Geometry check sheet. Reference: the model listing, model coordinates, mm. Face numbers are marked on the shaded views. A direction names the side the tool comes from. Coordinates: 2 decimals unless noted, no trailing zeros. Write each loop counter-clockwise with the first axis right and the second up, starting at its lowest first coordinate (ties: lowest second). Pieces come first, ordered by that corner, then holes. Notation, with made-up numbers: (61.25, 15) -> (101.25, 15) arc R26 ccw to (101.25, 39) -> close; hole circle Ø2 at (68.25, -25). An arc over 180 degrees is marked (long way). Use a Markdown table: item, result.
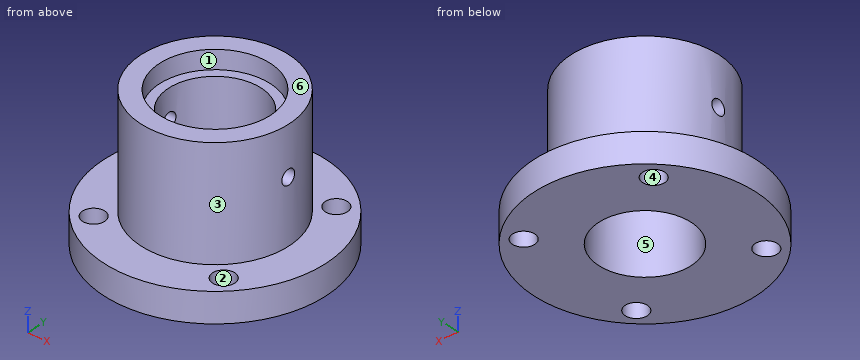
```python
from build123d import *

# Parameters (mm, degrees)
SKETCH_2_R          = 15
CUT_EXTRUDE_1_DEPTH = 5
SKETCH_3_R          = 12.5
CUT_EXTRUDE_2_DEPTH = 57.956123464
SKETCH_5_R          = 3
CUT_EXTRUDE_5_DEPTH = 57.956123464
SKETCH_6_R          = 2
CUT_EXTRUDE_6_DEPTH = 61


with BuildPart() as part:
    # 草图1 → 旋转1 (revolve)
    with BuildSketch(Plane(origin=(0, 0, 0), x_dir=(1, 0, 0), z_dir=(0, 1, 0)), mode=Mode.PRIVATE) as revolve_1_sk:
        Polygon((0, 0), (30, 0), (30, -8), (20, -8), (20, -38), (0, -38), align=None)
    revolve(revolve_1_sk.sketch.rotate(Axis((0, 0, 0), (0, 0, 1)), 180), axis=Axis((0, 0, 0), (0, 0, 1)))

    # 草图2 → 切除-拉伸1 (cut)
    with BuildSketch(Plane.XY.offset(38)):
        Circle(SKETCH_2_R)
    extrude(amount=-CUT_EXTRUDE_1_DEPTH, mode=Mode.SUBTRACT)

    # 草图3 → 切除-拉伸2 (cut, through all)
    with BuildSketch(Plane.XY.offset(38)):
        Circle(SKETCH_3_R)
    extrude(amount=-CUT_EXTRUDE_2_DEPTH, mode=Mode.SUBTRACT)

    # 草图5 → 切除-拉伸5 (cut, through all)
    with BuildSketch(Plane.XY):
        with Locations(Location((17.67767, 17.67767, 0), (0, 0, 180))):
            Circle(SKETCH_5_R)
        with Locations(Location((-17.67767, 17.67767, 0), (0, 0, 180))):
            Circle(SKETCH_5_R)
        with Locations(Location((-17.67767, -17.67767, 0), (0, 0, 180))):
            Circle(SKETCH_5_R)
        with Locations(Location((17.67767, -17.67767, 0), (0, 0, 180))):
            Circle(SKETCH_5_R)
    extrude(amount=CUT_EXTRUDE_5_DEPTH, mode=Mode.SUBTRACT)

    # 草图6 → 切除-拉伸6 (cut, symmetric)
    with BuildSketch(Plane(origin=(0, 0, 0), x_dir=(0, 0, -1), z_dir=(1, 0, 0))):
        with Locations((-25, 0)):
            Circle(SKETCH_6_R)
    extrude(amount=CUT_EXTRUDE_6_DEPTH, both=True, mode=Mode.SUBTRACT)


solid = part.part
```
Item 1: Thickness scan on L1, parallel to Z at x = 17, y = 0; L2, parallel to Y at x = 0, z = 34; L3, parallel to Y at x = 0, z = 25.5. Record the ranges inside material, lowest first. Write a range as [from, to].
Answer block:
| item | result |
|---|---|
| L1 | z = [0, 23], [27, 38] |
| L2 | y = [-20, -15], [15, 20] |
| L3 | y = [-20, -12.5], [12.5, 20] |
Item 2: Section check C-C on z = 25. Record the boundary of the cut face in (x, y).
Answer block:
| item | result |
|---|---|
| outline | (-19.9, -2) arc R20 ccw to (19.9, -2) -> (12.34, -2) arc R12.5 cw to (-12.34, -2) -> close; (-19.9, 2) -> (-12.34, 2) arc R12.5 cw to (12.34, 2) -> (19.9, 2) arc R20 ccw to start |
Item 3: Section check A-A on x = 0. Record the boundary of the cut face in (y, z), then the cut area to 3 significant figures.
Answer block:
| item | result |
|---|---|
| outline | (-30, 0) -> (-12.5, 0) -> (-12.5, 33) -> (-15, 33) -> (-15, 38) -> (-20, 38) -> (-20, 8) -> (-30, 8) -> close; (12.5, 0) -> (30, 0) -> (30, 8) -> (20, 8) -> (20, 38) -> (15, 38) -> (15, 33) -> (12.5, 33) -> close |
| area | 705 mm^2 |
Item 4: Tool access check on the marked faces 1 and 2. Record the directions out of +Z, -Z, +X, -X, +Y, -Y that give a thin tool (end or side, any length) a straight path to the whole face; none if there is none.
Answer block:
| item | result |
|---|---|
| face 1 | +Z |
| face 2 | +Z, -Z |
Item 5: Depth check by flat-ended pin: P1, Ø5, axis at y = 18, z = 32, coming from the -X side; P2, Ø1, axis at y = -4, z = 30, coming from the +X side; P3, Ø3.5, axis at x = -17.68, y = -17.68, coming from the -Z side; P4, Ø4.5, axis at y = 0, z = 25, coming from the -X side. Enter the tip coordinate at first touch or a pass-through.
Answer block:
| item | result |
|---|---|
| P1 | stops at x = -12.64 |
| P2 | stops at x = 19.69 |
| P3 | passes through |
| P4 | stops at x = -20 |
Item 6: Mould release check, pull along X, two halves, no side actions. Record for the marked faces 3, 4, 5 and 6: +X half, -X half, draft (parallel to the pull), parting line (faces both ways), or undercut.
Answer block:
| item | result |
|---|---|
| face 3 | parting line |
| face 4 | undercut |
| face 5 | undercut |
| face 6 | draft |
Item 7: Section check D-D on y = -7.5. Record the boundary of the cut face in (x, z), then the cut area to 3 significant figures.
Answer block:
| item | result |
|---|---|
| outline | (-29.05, 0) -> (-10, 0) -> (-10, 33) -> (-12.99, 33) -> (-12.99, 38) -> (-18.54, 38) -> (-18.54, 8) -> (-29.05, 8) -> close; (10, 0) -> (29.05, 0) -> (29.05, 8) -> (18.54, 8) -> (18.54, 38) -> (12.99, 38) -> (12.99, 33) -> (10, 33) -> close |
| area | 787 mm^2 |
Item 8: Section check B-B on y = 0. Record the boundary of the cut face in (x, z), then the cut area to 3 significant figures.
Answer block:
| item | result |
|---|---|
| outline | (-30, 0) -> (-12.5, 0) -> (-12.5, 23) -> (-20, 23) -> (-20, 8) -> (-30, 8) -> close; (-20, 27) -> (-12.5, 27) -> (-12.5, 33) -> (-15, 33) -> (-15, 38) -> (-20, 38) -> close; (12.5, 0) -> (30, 0) -> (30, 8) -> (20, 8) -> (20, 23) -> (12.5, 23) -> close; (12.5, 27) -> (20, 27) -> (20, 38) -> (15, 38) -> (15, 33) -> (12.5, 33) -> close |
| area | 645 mm^2 |
